```python
from build123d import *

# Parameters (mm, degrees)
F1_DEPTH = 50.8
F3_DEPTH = 10.4902
F5_DEPTH = 10.4902
F6_W     = 24.436295
F6_H     = 29.8196
F7_DEPTH = 2.032


with BuildPart() as f1:
    # F0 (on Front) → F1 (new body)
    with BuildSketch(Plane.XZ):
        Polygon((0, 87.4776), (0, 0), (101.473, 0), (101.473, 59.4868), (51.991789, 108.968011), (39.748989, 108.968011), (18.258578, 87.4776), align=None)
    extrude(amount=F1_DEPTH)

    # F2 (on face) → F3 (cut)
    with BuildSketch(Plane.XZ.offset(50.8)):
        Polygon((21.27824, 87.479748), (21.27824, 90.497263), (18.258578, 87.4776), align=None)
        Polygon((24.362021, 90.497263), (24.362021, 93.581043), (21.27824, 90.497263), align=None)
        Polygon((27.44224, 93.581043), (27.44224, 96.661262), (24.362021, 93.581043), align=None)
        Polygon((30.520708, 96.661262), (30.520708, 99.73973), (27.44224, 96.661262), align=None)
        Polygon((33.59858, 99.73973), (33.59858, 102.817602), (30.520708, 99.73973), align=None)
        Polygon((36.676452, 102.817602), (36.676452, 105.895475), (33.59858, 102.817602), align=None)
        Polygon((39.748989, 105.895475), (39.748989, 108.968011), (36.676452, 105.895475), align=None)
    extrude(amount=-F3_DEPTH, mode=Mode.SUBTRACT)

    # F4 (on face) → F5 (cut)
    with BuildSketch(Plane(origin=(0, 0, 0), x_dir=(-1, 0, 0), z_dir=(0, 1, 0))):
        Polygon((-36.672943, 105.891965), (-39.748989, 108.968011), (-39.748989, 105.891965), align=None)
        Polygon((-18.258578, 87.4776), (-21.280885, 90.499908), (-21.280885, 87.4776), align=None)
        Polygon((-21.280885, 90.499908), (-24.358757, 93.57778), (-24.358757, 90.499908), align=None)
        Polygon((-24.358757, 93.57778), (-27.439327, 96.658349), (-27.439327, 93.57778), align=None)
        Polygon((-27.439327, 96.658349), (-30.517199, 99.736221), (-30.517199, 96.658349), align=None)
        Polygon((-30.517199, 99.736221), (-33.595071, 102.814093), (-33.595071, 99.736221), align=None)
        Polygon((-33.595071, 102.814093), (-36.672943, 105.891965), (-36.672943, 102.814093), align=None)
    extrude(amount=-F5_DEPTH, mode=Mode.SUBTRACT)

    # F6 (on face) → F7 (join)
    with BuildSketch(Plane.XY.offset(87.4776)):
        with Locations((12.218147, -25.4)):
            Rectangle(F6_W, F6_H)
    extrude(amount=F7_DEPTH)


solid = f1.part
```
Geometry: final body of the model. Coordinates: model frame, mm. A direction names the side the tool comes from. Round coordinates to 2 decimals unless told otherwise and drop trailing zeros. Write each loop counter-clockwise with the first axis right and the second up, starting at its lowest first coordinate (ties: lowest second). Pieces come first, ordered by that corner, then holes.
Item 1: Section query B-B (x = 7). Return loops of the section in (y, z), plus the area to 3 significant figures.
Item 2: Pin query (flat end, axial travel): P1, Ø1.5, axis at y = -44, z = 95.5, coming from the -X side; P2, Ø2, axis at x = 26.5, y = -15.5, coming from the -Z side; P3, Ø2.5, axis at x = 26, z = 95.5, coming from the +Y side; P4, Ø2.5, axis at x = 28.5, y = -46, coming from the +Z side. Return the tip coordinate at first contact, or that it passes through.
Item 3: Material intervals for L1, parallel to Z at x = 15.5, y = -39; L2, parallel to X at y = -26, z = 75; L3, parallel to X at y = -23, z = 93.5, sorted ascending.
Item 4: Set-up query: faces 1 (the face through (21.281, -5, 89)), 2 (the face through (30.16, -25.04, 99.38)), 3 (the face through (38, -46, 105.895)). Return all of +Z, -Z, +X, -X, +Y, -Y with unobstructed straight access to the full face (end or side cutting, diameter ignored); none if empty.
Completed:
1. outline: (-50.8, 0) - (0, 0) - (0, 87.48) - (-10.49, 87.48) - (-10.49, 89.51) - (-40.31, 89.51) - (-40.31, 87.48) - (-50.8, 87.48) - close
1. area: 4,500 mm2
2. P1: stops at x = 27.44
2. P2: stops at z = 0
2. P3: stops at y = -10.49
2. P4: stops at z = 96.66
3. L1: z = 0 to 89.51
3. L2: x = 0 to 85.96
3. L3: x = 24.28 to 67.46
4. face 1: +Z, -X, +Y
4. face 2: +Z, -X, +Y, -Y
4. face 3: +Z, -X, -Y
